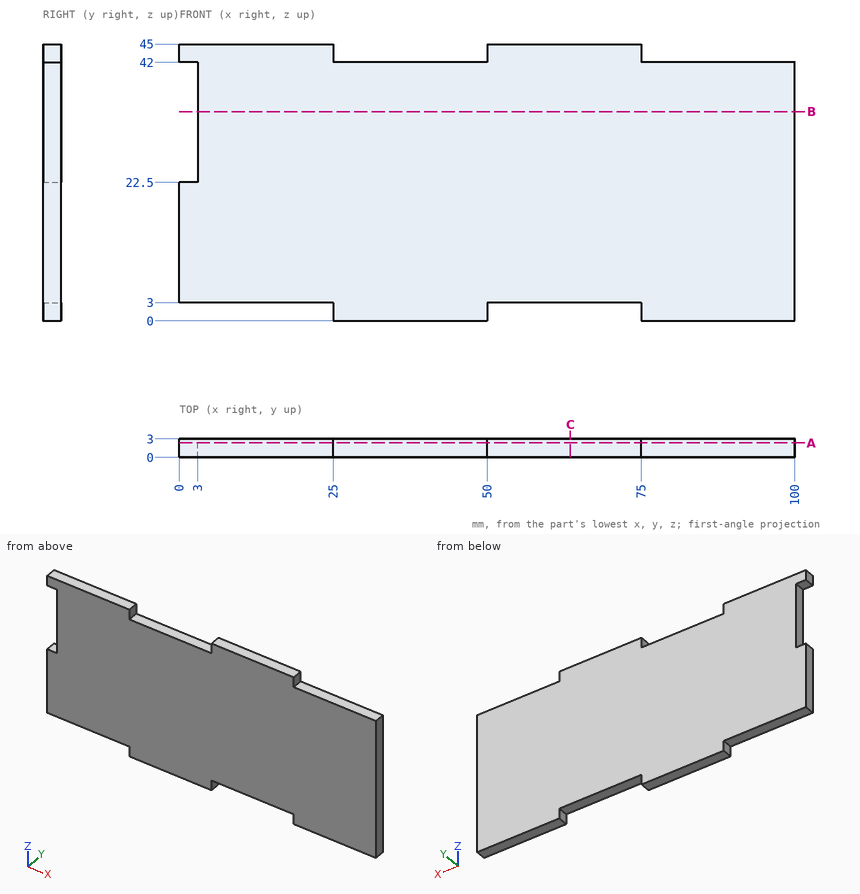
Geometry: see drawing. Coordinates: mm, zero at the bounding-box minimum. Round coordinates to 2 decimals unless told otherwise and drop trailing zeros. Write each loop counter-clockwise with the first axis right and the second up, starting at its lowest first coordinate (ties: lowest second). Pieces come first, ordered by that corner, then holes.
1) Ray query, L1, parallel to Z at x = 39, y = 2.5; L2, parallel to Z at x = 60.5, y = 0.4; L3, parallel to X at y = 1.8, z = 32. Return the intervals inside material, ascending.
2) Cut plane C-C (x = 63.5). Return the cut outline in (y, z).
3) Cut plane A-A (y = 2.35). Return the cut outline in (x, z), then the cut area to 3 significant figures.
4) Contact query for flat-ended pins moving along their axis: P1, Ø1.5, axis at y = 1, z = 43.5, coming from the +X side; P2, Ø0.9, axis at x = 2, y = 1, coming from the -Z side; P3, Ø0.9, axis at y = 1, z = 1.5, coming from the -X side. Output: stop coordinate, or through.
5) Cut plane B-B (z = 34). Return the cut outline in (x, y).
Geometry says:
1. L1: z = 0 to 42
1. L2: z = 3 to 45
1. L3: x = 3 to 100
2. outline: (0, 3) - (3, 3) - (3, 45) - (0, 45) - close
3. outline: (0, 3) - (25, 3) - (25, 0) - (50, 0) - (50, 3) - (75, 3) - (75, 0) - (100, 0) - (100, 42) - (75, 42) - (75, 45) - (50, 45) - (50, 42) - (25, 42) - (25, 45) - (0, 45) - (0, 42) - (3, 42) - (3, 22.5) - (0, 22.5) - close
3. area: 4,140 mm2
4. P1: stops at x = 75
4. P2: stops at z = 3
4. P3: stops at x = 25
5. outline: (3, 0) - (100, 0) - (100, 3) - (3, 3) - close
